Autodesk Inventor part; units mm, degrees
ref_plane "YZ Plane" through (0, 0, 0) normal (1, 0, 0) x (0, 1, 0)
ref_plane "XZ Plane" through (0, 0, 0) normal (0, 1, 0) x (-1, 0, 0)
ref_plane "XY Plane" through (0, 0, 0) normal (0, 0, 1) x (1, 0, 0)
sketch "Sketch1" plane through (0, 0, 0) normal (0, 0, 1) x (1, 0, 0)
  line L0 (0, 0) -> (50, 0)
  line L1 (50, 0) -> (50, -15)
  line L2 (50, -15) -> (0, -15)
  line L3 (0, -15) -> (0, 0)
  line L4 (0, 0) -> (15, -15)
  line L5 (0, 0) -> (21.2132, 0) construction
  circle A0 centre (7.5, -7.5) radius 4.05
  line L6 (50, 0) -> (35, -15)
  circle A1 centre (42.5, -7.5) radius 4.05
  circle A2 centre (25, -7) radius 2.65
  circle A3 centre (7.5, -7.5) radius 7.5
  circle A4 centre (42.5, -7.5) radius 7.5
  line L7 (25, -7) -> (25, 0)
  point P0 (0, 0)
  dimension "d0" = 50
  dimension "d1" = 15
  dimension "d2" = 45
  dimension "d3" = 8.1
  dimension "d4" = 8.1
  dimension "d5" = 45
  dimension "d9" = 0
  dimension "d13" = 0
  dimension "d14" = 5.3
  dimension "d18" = 7
  dimension "d19" = 25
  dimension "d20" = 0
extrude "Extrusion1" add sketch "Sketch1" along normal blind 15 contours L4 A3 L3 | L0 A3 L4 | L0 A4 L6 L2 L4 A3 | A3 L4 A0 | A3 L2 L3 | A3 L4 A0 | A3 L4 L2 | L0 L6 A4 | A4 L6 A1 | L1 A4 L6 | A4 L6 A1 | A4 L2 L6 | L1 L2 A4
fillet "Fillet1" radius 2 4 edges at (50, -15, 7.5) (50, 0, 7.5) (0, -15, 7.5) (0, 0, 7.5)
properties part number "Support_Seperator(Middle rod)"
Check sheet for the modelled part. Datum: model origin and axes. Units: mm. Give positions to 0.01 mm unless a question says otherwise; leave off trailing zeros. Loops run counter-clockwise (first coordinate to the right, second up) from the corner with the lowest first, then second, coordinate; pieces in that order, holes last. Notation, with made-up numbers: (54, -33.75) - (84, -33.75) arc R32 cw to (84, 0.25) - close; hole circle Ø3 at (35, 72). An arc over 180 degrees is marked (long way). One line per question, with ' | ' between items. Start each with the question number.
1. Cross-section at B-B, the plane z = 11.25. Enter the section's corners in (x, y).
2. Material ranges on line 1 along X through (y, z) = (-9.25, 7.75); line 2 along X through (y, z) = (-5.75, 12); line 3 along Y through (x, z) = (25, 8.5), recorded low to high. Write a range as [from, to].
3. Cross-section at D-D, the plane y = -7. Enter the section's corners in (x, z), plus the area to 3 significant figures.
4. Cross-section at A-A, the plane x = 42.5. Enter the section's corners in (y, z), plus the area to 4 significant figures.
5. Cross-section at C-C, the plane y = -11. Enter the section's corners in (x, z), plus the area to 3 significant figures.
6. Draft check along Y on faces 1 (the cylindrical face through (9.7, -10.9, 7.4)), 2 (the flat face through (0, -8, 7)), 3 (the cylindrical face through (49.4, -14.43, 7.6)). Enter one of: released by +Y, released by -Y, zero draft, split by the parting line, or undercut.
Check result:
1) outline: (0, -13) arc R2 ccw to (2, -15) - (48, -15) arc R2 ccw to (50, -13) - (50, -2) arc R2 ccw to (48, 0) - (2, 0) arc R2 ccw to (0, -2) - close; hole circle Ø8.1 at (7.5, -7.5); hole circle Ø5.3 at (25, -7); hole circle Ø8.1 at (42.5, -7.5)
2) line 1: x = [0, 3.85], [11.15, 23.6], [26.4, 38.85], [46.15, 50] | line 2: x = [0, 3.85], [11.15, 22.66], [27.34, 38.85], [46.15, 50] | line 3: y = [-15, -9.65], [-4.35, 0]
3) outline: (0, 0) - (3.48, 0) - (3.48, 15) - (0, 15) - close; (11.52, 0) - (22.35, 0) - (22.35, 15) - (11.52, 15) - close; (27.65, 0) - (38.48, 0) - (38.48, 15) - (27.65, 15) - close; (46.52, 0) - (50, 0) - (50, 15) - (46.52, 15) - close | area: 429 mm2
4) outline: (-15, 0) - (-11.55, 0) - (-11.55, 15) - (-15, 15) - close; (-3.45, 0) - (0, 0) - (0, 15) - (-3.45, 15) - close | area: 103.5 mm2
5) outline: (0, 0) - (5.46, 0) - (5.46, 15) - (0, 15) - close; (9.54, 0) - (40.46, 0) - (40.46, 15) - (9.54, 15) - close; (44.54, 0) - (50, 0) - (50, 15) - (44.54, 15) - close | area: 628 mm2
6) face 1: undercut | face 2: zero draft | face 3: released by -Y
